from build123d import *

# Parameters (mm, degrees)
SKETCH1_R           = 2.413
BOSS_EXTRUDE1_DEPTH = 44.45
SKETCH2_R           = 2.413
CUT_EXTRUDE1_DEPTH  = 50.8


with BuildPart() as part:
    # Sketch1 → Boss-Extrude1 (new body)
    with BuildSketch(Plane(origin=(0, 0, 0), x_dir=(1, 0, 0), z_dir=(0, 1, 0))):
        Polygon((0, 38.1), (6.35, 44.45), (38.1, 44.45), (44.45, 38.1), (44.45, 6.35), (38.1, 0), (6.35, 0), (0, 6.35), align=None)
        with Locations((9.525, 22.225)):
            Circle(SKETCH1_R, mode=Mode.SUBTRACT)
        with Locations((22.225, 22.225)):
            Circle(SKETCH1_R, mode=Mode.SUBTRACT)
        with Locations((34.925, 22.225)):
            Circle(SKETCH1_R, mode=Mode.SUBTRACT)
    extrude(amount=BOSS_EXTRUDE1_DEPTH)

    # Sketch2 → Cut-Extrude1 (cut)
    with BuildSketch(Plane(origin=(44.45, 0, 0), x_dir=(0, 0, -1), z_dir=(1, 0, 0))):
        with Locations((9.525, 31.75)):
            Circle(SKETCH2_R)
        with Locations((34.925, 31.75)):
            Circle(SKETCH2_R)
        with Locations((34.925, 6.35)):
            Circle(SKETCH2_R)
        with Locations((9.525, 6.35)):
            Circle(SKETCH2_R)
        with Locations((9.525, 19.05)):
            Circle(SKETCH2_R)
        with Locations((34.925, 19.05)):
            Circle(SKETCH2_R)
    extrude(amount=-CUT_EXTRUDE1_DEPTH, mode=Mode.SUBTRACT)


solid = part.part
Read the model definition and answer for the solid it produces. Units are mm, in the model's axes. Round coordinates to 2 decimals unless told otherwise and drop trailing zeros. Write each loop counter-clockwise with the first axis right and the second up, starting at its lowest first coordinate (ties: lowest second). Pieces come first, ordered by that corner, then holes. Notation, with made-up numbers: (64.25, 45) - (102.25, 45) arc R7 ccw to (102.25, 58) - close; hole circle Ø4 at (-24, 30.5). An arc over 180 degrees is marked (long way). One line per question, with ' | ' between items. Start each with the question number.
1. Section C-C (z = -34.5) is taken. Determine the outline of the cut face in (x, y).
2. Section B-B (x = 36) is taken. Determine the outline of the cut face in (y, z) (3 decimals), and give its area (3 significant figures).
3. Section D-D (x = 5.5) is taken. Determine the outline of the cut face in (y, z) (3 decimals).
4. Find the intervals of material crossed by probe 1 along Z at (x, y) = (5, 20.5); probe 2 along Y at (x, z) = (35.5, -9.5); probe 3 along X at (y, z) = (32.5, -21.5), in increasing order. Write a range as [from, to].
5. Section A-A (y = 6.35) is taken. Determine the outline of the cut face in (x, z) (3 decimals), and give its area (3 significant figures).
6. For a pull along Z with two mould halves and no side action, classify faces 1 (the face through (41.23, 21.91, -41.32)), 2 (the face through (22.536, 19.156, -32.514)), 3 (the face through (27, 0, -23)) as +Z half, -Z half, draft (parallel to the pull), parting line (faces both ways), or undercut.
7. This flat-tipped pin is pushed along its axis until it touches: pin 1 (4 mm diameter, centred on y = 6.35, z = -34.925, fed in from +X). Where does it stop, or does it pass through?
Filled in:
1) outline: (0, 0) - (44.45, 0) - (44.45, 3.97) - (0, 3.97) - close; (0, 8.73) - (44.45, 8.73) - (44.45, 16.67) - (0, 16.67) - close; (0, 21.43) - (44.45, 21.43) - (44.45, 29.37) - (0, 29.37) - close; (0, 34.13) - (44.45, 34.13) - (44.45, 44.45) - (0, 44.45) - close
2) outline: (0, -44.45) - (44.45, -44.45) - (44.45, -24.385) - (0, -24.385) - close; (0, -20.065) - (44.45, -20.065) - (44.45, 0) - (0, 0) - close; hole circle Ø4.826 at (6.35, -34.925); hole circle Ø4.826 at (6.35, -9.525); hole circle Ø4.826 at (19.05, -34.925); hole circle Ø4.826 at (19.05, -9.525); hole circle Ø4.826 at (31.75, -34.925); hole circle Ø4.826 at (31.75, -9.525) | area: 1,670 mm²
3) outline: (0, -43.6) - (44.45, -43.6) - (44.45, -0.85) - (0, -0.85) - close; hole circle Ø4.826 at (6.35, -34.925); hole circle Ø4.826 at (6.35, -9.525); hole circle Ø4.826 at (19.05, -34.925); hole circle Ø4.826 at (19.05, -9.525); hole circle Ø4.826 at (31.75, -34.925); hole circle Ø4.826 at (31.75, -9.525)
4) probe 1: [-43.1, -36.85], [-33, -11.45], [-7.6, -1.35] | probe 2: [0, 3.94], [8.76, 16.64], [21.46, 29.34], [34.16, 44.45] | probe 3: [0, 7.22], [11.83, 19.92], [24.53, 32.62], [37.23, 44.45]
5) outline: (0, -38.1) - (6.35, -44.45) - (38.1, -44.45) - (44.45, -38.1) - (44.45, -37.338) - (0, -37.338) - close; (0, -32.512) - (44.45, -32.512) - (44.45, -11.938) - (0, -11.938) - close; (0, -7.112) - (44.45, -7.112) - (44.45, -6.35) - (38.1, 0) - (6.35, 0) - (0, -6.35) - close; hole circle Ø4.826 at (9.525, -22.225); hole circle Ø4.826 at (22.225, -22.225); hole circle Ø4.826 at (34.925, -22.225) | area: 1,410 mm²
6) face 1: -Z half | face 2: undercut | face 3: draft
7) pin 1: through
